from build123d import *
from build123d.topology import SkipClean

# Parameters (mm, degrees)
BOSS_EXTRUDE1_DEPTH     = 590
SKETCH2_R               = 25
BOSS_EXTRUDE2_DEPTH     = 650
SKETCH2_4_R             = 225
CUT_EXTRUDE2_DEPTH      = 1236.329432749
CUT_EXTRUDE4_DEPTH      = 1624.31086661
CUT_EXTRUDE4_DEPTH_BACK = 1624.31086661
SKETCH3_W               = 86.663012773
SKETCH3_H               = 630


with BuildPart() as part:
    # Sketch1 → Boss-Extrude1 (new body)
    with BuildSketch(Plane.XY):
        with BuildLine():
            Line((-542, 645), (-542, 0))
            Line((-542, 0), (-125, 0))
            Line((-125, 0), (-125, 99.927755898))
            ThreePointArc((-125, 99.927755898), (0, 224.927755898), (125, 99.927755898))
            Line((125, 99.927755898), (125, 0))
            Line((125, 0), (542, 0))
            Line((542, 0), (542, 645))
            Line((542, 645), (150, 645))
            Line((150, 645), (150, 400))
            Line((150, 400), (-150, 400))
            Line((-150, 400), (-150, 645))
            Line((-150, 645), (-542, 645))
        make_face()
        Polygon((-542, 645), (-769.142885948, 645), (-769.142885948, 650), (769.142885948, 650), (769.142885948, 645), (542, 645), align=None)
    extrude(amount=BOSS_EXTRUDE1_DEPTH)

    # Sketch2 → Boss-Extrude2 (add)
    # profile 1 of 6: a face of its own
    with BuildSketch(Plane(origin=(0, 650, 0), x_dir=(1, 0, 0), z_dir=(0, 1, 0))):
        Polygon((-541.5, 86.663012773), (-541.5, 0), (-244.996182612, 0), (-244.996182612, 86.663012773), (-274.996182612, 116.663012773), (-511.5, 116.663012773), align=None)
        with Locations(Location((-312.5, 71.663012773, 0), (0, 0, 270))):
            Circle(SKETCH2_R, mode=Mode.SUBTRACT)
    # profile 2 of 6: a face of its own
    with BuildSketch(Plane(origin=(0, 650, 0), x_dir=(1, 0, 0), z_dir=(0, 1, 0))):
        with BuildLine():
            Line((-100, 125.512423659), (-244.996182612, 0))
            Line((-244.996182612, 0), (-75, 0))
            ThreePointArc((-75, 0), (0, 75), (75, 0))
            Line((75, 0), (244.996182612, 0))
            Line((244.996182612, 0), (100, 125.512423659))
            Line((100, 125.512423659), (-100, 125.512423659))
        make_face()
    # profile 3 of 6: a face of its own
    with BuildSketch(Plane(origin=(0, 650, 0), x_dir=(1, 0, 0), z_dir=(0, 1, 0))):
        Polygon((244.996182612, 86.663012773), (244.996182612, 0), (541.5, 0), (541.5, 86.663012773), (511.5, 116.663012773), (274.996182612, 116.663012773), align=None)
        with Locations(Location((312.5, 71.663012773, 0), (0, 0, 270))):
            Circle(SKETCH2_R, mode=Mode.SUBTRACT)
    # profile 4 of 6: a face of its own
    with BuildSketch(Plane(origin=(0, 650, 0), x_dir=(1, 0, 0), z_dir=(0, 1, 0))):
        Polygon((541.5, -590), (244.996182612, -590), (244.996182612, -676.663012773), (274.996182612, -706.663012773), (511.5, -706.663012773), (541.5, -676.663012773), align=None)
        with Locations(Location((312.5, -661.663012773, 0), (0, 0, 270))):
            Circle(SKETCH2_R, mode=Mode.SUBTRACT)
    # profile 5 of 6: a face of its own
    with BuildSketch(Plane(origin=(0, 650, 0), x_dir=(1, 0, 0), z_dir=(0, 1, 0))):
        with BuildLine():
            Line((-75, -590), (-244.996182612, -590))
            Line((-244.996182612, -590), (-100, -715.512423659))
            Line((-100, -715.512423659), (100, -715.512423659))
            Line((100, -715.512423659), (244.996182612, -590))
            Line((244.996182612, -590), (75, -590))
            ThreePointArc((75, -590), (0, -665), (-75, -590))
        make_face()
    # profile 6 of 6: a face of its own
    with BuildSketch(Plane(origin=(0, 650, 0), x_dir=(1, 0, 0), z_dir=(0, 1, 0))):
        Polygon((-244.996182612, -590), (-541.5, -590), (-541.5, -676.663012773), (-511.5, -706.663012773), (-274.996182612, -706.663012773), (-244.996182612, -676.663012773), align=None)
        with Locations(Location((-312.5, -661.663012773, 0), (0, 0, 270))):
            Circle(SKETCH2_R, mode=Mode.SUBTRACT)
    extrude(amount=-BOSS_EXTRUDE2_DEPTH)

    # Sketch2_4 → Cut-Extrude2 (cut, through all)
    with SkipClean():  # the faces are left unmerged after this step: merging them gives an invalid solid
        with BuildSketch(Plane(origin=(0, 650, 0), x_dir=(1, 0, 0), z_dir=(0, 1, 0))):
            with Locations(Location((-455.251684993, -295, 0), (0, 0, 270))):
                Circle(SKETCH2_4_R)
            with Locations(Location((455.251684993, -295, 0), (0, 0, 270))):
                Circle(SKETCH2_4_R)
            with BuildLine():
                ThreePointArc((75, -590), (0, -515), (-75, -590))
                Line((-75, -590), (75, -590))
            make_face()
            with BuildLine():
                Line((75, -590), (-75, -590))
                ThreePointArc((-75, -590), (0, -665), (75, -590))
            make_face()
            with BuildLine():
                ThreePointArc((75, 0), (0, 75), (-75, 0))
                Line((-75, 0), (75, 0))
            make_face()
            with BuildLine():
                Line((75, 0), (-75, 0))
                ThreePointArc((-75, 0), (0, -75), (75, 0))
            make_face()
            with BuildLine():
                ThreePointArc((-541.5, -590), (-762.601277219, -295), (-541.5, 0))
                Line((-541.5, 0), (-769.142885948, 0))
                Line((-769.142885948, 0), (-769.142885948, -590))
                Line((-769.142885948, -590), (-541.5, -590))
            make_face()
            with BuildLine():
                Line((769.142885948, 0), (541.5, 0))
                ThreePointArc((541.5, 0), (762.601277219, -295), (541.5, -590))
                Line((541.5, -590), (769.142885948, -590))
                Line((769.142885948, -590), (769.142885948, 0))
            make_face()
        extrude(amount=-CUT_EXTRUDE2_DEPTH, mode=Mode.SUBTRACT)

    # Sketch3 → Cut-Extrude4 (cut, two sides: drawn at the far end of the back side and taken through both)
    with BuildSketch(Plane(origin=(541.5, 0, 0), x_dir=(0, 0, -1), z_dir=(1, 0, 0)).offset(-CUT_EXTRUDE4_DEPTH_BACK)):
        Polygon((-864.95540651, 20), (-716.879953267, 20), (-590, 20), (-590, 650), (-864.95540651, 650), align=None)
        Polygon((176.90498613, 650), (86.663012773, 650), (86.663012773, 20), (151.95407612, 20), (176.90498613, 20), align=None)
        with Locations((43.331506387, 335)):
            Rectangle(SKETCH3_W, SKETCH3_H)
        Polygon((-570, 630), (-570, 0), (-570, -112.404091098), (-20, -112.404091098), (-20, 0), (-20, 630), align=None)
    extrude(amount=CUT_EXTRUDE4_DEPTH + CUT_EXTRUDE4_DEPTH_BACK, mode=Mode.SUBTRACT)


solid = part.part
Can you work these out from the model? Positions are in its coordinate system, mm. A direction names the side the tool comes from. Coordinates: 2 decimals unless noted, no trailing zeros. Write each loop counter-clockwise with the first axis right and the second up, starting at its lowest first coordinate (ties: lowest second). Pieces come first, ordered by that corner, then holes.
Q1. Imagine slicing it at C-C, the plane x = -16. List the corners of the cut face in (y, z) for me, plus the area to 3 significant figures.
Results found:
outline: (0, -125.51) - (20, -125.51) - (20, -73.27) - (0, -73.27) - close; (0, 663.27) - (20, 663.27) - (20, 715.51) - (0, 715.51) - close; (645, 73.27) - (650, 73.27) - (650, 516.73) - (645, 516.73) - close
area: 4,310 mm2
Q2. Imagine slicing it at A-A, the plane z = 295. List the corners of the cut face in (x, y) for me, plus the area to 3 significant figures.
Results found:
outline: (-762.6, 645) - (-680.25, 645) - (-680.25, 650) - (-762.6, 650) - close; (-230.25, 630) - (-150, 630) - (-150, 645) - (150, 645) - (150, 630) - (230.25, 630) - (230.25, 650) - (-230.25, 650) - close; (680.25, 645) - (762.6, 645) - (762.6, 650) - (680.25, 650) - close
area: 5,530 mm2
Q3. If we mould it in two halves opening along Z, with no side actions, what happens to faces 1 (the face through (-526.71, 10.14, 691.453)), 2 (the face through (-395, 20, 649)), 3 (the face through (255.638, 640.14, 398.824)), 4 (the face through (213, 630, 291))? For each: +Z half, -Z half, draft (parallel to the pull), parting line (faces both ways), or undercut.
Results found:
face 1: +Z half
face 2: draft
face 3: undercut
face 4: undercut
Q4. Imagine slicing it at B-B, the plane y = 465. List the corners of the cut face in (x, z) for me, plus the area to 3 significant figures.
Results found:
outline: (-542, 0.15) arc R307.35 ccw to (-541.5, 0) - (-150, 0) - (-150, 20) - (-542, 20) - close; (-542, 570) - (-150, 570) - (-150, 590) - (-541.5, 590) arc R307.35 ccw to (-542, 589.85) - close; (150, 0) - (541.5, 0) arc R307.35 ccw to (542, 0.15) - (542, 20) - (150, 20) - close; (150, 570) - (542, 570) - (542, 589.85) arc R307.35 ccw to (541.5, 590) - (150, 590) - close
area: 31,400 mm2
Q5. For P1, Ø10, axis at x = -378.5, y = 6.5, coming from the -Z side; P2, Ø4, axis at x = -408.5, y = 143, coming from the +Z side; P3, Ø10, axis at y = 37.5, z = 14.5, coming from the +X side, each with a flat end and sliding along its axis, tell me the tip position at first contact or that it passes through.
Results found:
P1: stops at z = -116.66
P2: stops at z = 590
P3: stops at x = 542
Q6. Which directions (+Z, -Z, +X, -X, +Y, -Y) give clear straight access to the entire face, cutting with the end or side of a thin tool? Please do faces 5 (the face through (259.786, 10.14, 691.453)), 6 (the face through (-111.423, 156.585, 579.86)), 7 (the face through (391, 20, -58)), 8 (the face through (703, 645, 291)).
Results found:
face 5: +Z, +Y, -Y
face 6: +Z, -Z, -Y
face 7: -Z, +X, -X, +Y
face 8: +Z, -Z, +X, -Y
Q7. Please list where these lines run through material, in increasing order: L1, parallel to X at y = 643.5, z = 295; L2, parallel to Z at x = 419, y = 136; L3, parallel to X at y = 102, z = 579.
Results found:
L1: x = -230.25 to -150, 150 to 230.25
L2: z = 0 to 20, 570 to 590
L3: x = -542 to -124.98, 124.98 to 542
Q8. Imagine slicing it at D-D, the plane z = 555. List the corners of the cut face in (x, y) for me, plus the area to 3 significant figures.
Results found:
outline: (-619.15, 645) - (-542, 645) - (-542, 630) - (-150, 630) - (-150, 645) - (-66.33, 645) - (-66.33, 650) - (-619.15, 650) - close; (66.33, 645) - (150, 645) - (150, 630) - (542, 630) - (542, 645) - (619.15, 645) - (619.15, 650) - (66.33, 650) - close
area: 17,300 mm2
